The listing builds one solid part. Answer for the finished solid, in the listing's coordinates (mm). A direction names the side the tool comes from. Give positions to 0.01 mm unless a question says otherwise; leave off trailing zeros. Write each loop counter-clockwise with the first axis right and the second up, starting at its lowest first coordinate (ties: lowest second). Pieces come first, ordered by that corner, then holes. Notation, with made-up numbers: (35, 7.5) -> (45, 7.5) arc R26 cw to (45, 34.5) -> close; hole circle Ø10 at (59, 44). An arc over 180 degrees is marked (long way). Write each question's results on one line, items separated by ' | '. Start each with the question number.
from build123d import *

# Parameters (mm, degrees)
EXTRUDE1_DEPTH            = 12.7
F_6_32_TAPPED_HOLE3_D     = 2.7051
SKETCH14_R                = 1.85
CUT_EXTRUDE6_DEPTH        = 24.153833376
F_6_32_TAPPED_HOLE5_D     = 2.7051
F_6_32_TAPPED_HOLE5_DEPTH = 50.8
F_6_32_TAPPED_HOLE5_TIP   = 0.81269403
CUT_EXTRUDE26_DEPTH       = 6
SKETCH25_R                = 5.7
CUT_EXTRUDE27_DEPTH       = 23.907422501
SKETCH26_R                = 8
CUT_EXTRUDE28_DEPTH       = 6


with BuildPart() as part:
    # Sketch1 → Extrude1 (new body)
    with BuildSketch(Plane.XY):
        with BuildLine():
            Line((0, 0), (0, 0.5))
            Line((0, 0.5), (15.5, 0.5))
            Line((15.5, 0.5), (15.5, 4))
            ThreePointArc((15.5, 4), (11.819050527, 4.746581358), (8.719864541, 6.868330393))
            ThreePointArc((8.719864541, 6.868330393), (-11.1, 0), (8.719864541, -6.868330393))
            ThreePointArc((8.719864541, -6.868330393), (11.819050527, -4.746581358), (15.5, -4))
            Line((15.5, -4), (15.5, -0.5))
            Line((15.5, -0.5), (0, -0.5))
            Line((0, -0.5), (0, 0))
        make_face()
    extrude(amount=-EXTRUDE1_DEPTH)

    # #6-32 Tapped Hole3 (through all)
    with Locations(Plane(origin=(-5.656516225, 5.657192254, 0), x_dir=(1, 0, 0), z_dir=(0, 0, 1))):
        with Locations((0, 0), (11.313708479, -0.000676029), (11.31303245, -11.314384508), (-0.000676029, -11.313708479)):
            Hole(F_6_32_TAPPED_HOLE3_D / 2)

    # Sketch14 → Cut-Extrude6 (cut, through all)
    with BuildSketch(Plane.XZ.offset(-0.5)):
        with Locations(Location((13, -3.5, 0), (0, 0, 270))):
            Circle(SKETCH14_R)
    extrude(amount=-CUT_EXTRUDE6_DEPTH, mode=Mode.SUBTRACT)

    # #6-32 Tapped Hole5
    with Locations(Plane(origin=(0, -0.5, 0), x_dir=(-1, 0, 0), z_dir=(0, 1, 0))):
        with Locations((-13, -3.5)):
            Hole(F_6_32_TAPPED_HOLE5_D / 2, depth=F_6_32_TAPPED_HOLE5_DEPTH)
            with Locations((0, 0, -(F_6_32_TAPPED_HOLE5_DEPTH + F_6_32_TAPPED_HOLE5_TIP / 2))):  # 118° drill point
                Cone(0, F_6_32_TAPPED_HOLE5_D / 2, F_6_32_TAPPED_HOLE5_TIP, mode=Mode.SUBTRACT)

    # Sketch24 → Cut-Extrude26 (cut)
    with BuildSketch(Plane(origin=(15.5, 0, 0), x_dir=(0, 0, -1), z_dir=(1, 0, 0))):
        with BuildLine():
            Line((0.2, 4), (6.832300833, 4))
            ThreePointArc((6.832300833, 4), (3.516150417, 6.820400286), (0.2, 4))
        make_face()
    extrude(amount=-CUT_EXTRUDE26_DEPTH, mode=Mode.SUBTRACT)

    # Sketch25 → Cut-Extrude27 (cut, through all)
    with BuildSketch(Plane.XY):
        Circle(SKETCH25_R)
    extrude(amount=-CUT_EXTRUDE27_DEPTH, mode=Mode.SUBTRACT)

    # Sketch26 → Cut-Extrude28 (cut)
    with BuildSketch(Plane.XY):
        Circle(SKETCH26_R)
    extrude(amount=-CUT_EXTRUDE28_DEPTH, mode=Mode.SUBTRACT)


solid = part.part
1. The mould has two halves that part along X. Classify faces 6 (the flat face through (11, -0.5, -6)), 7 (the cylindrical face through (-8, 0, -3)), 8 (the cylindrical face through (11.77, -4.767, -6.261)): pulls with the +X half, pulls with the -X half, needs draft (parallel to the pull), parting line crosses it, or undercut.
2. Consider probe 1 along X at (y, z) = (1.5, -5); probe 2 along X at (y, z) = (-2, -3.5); probe 3 along Y at (x, z) = (-0.75, -4.25). Determine where each line is inside the solid, lowest interval first. Write a range as [from, to].
3. Section D-D (z = -11) is taken. Write down the section's boundary in (x, y), then the cut area to 3 significant figures.
4. Section A-A (y = 3.25) is taken. Write down the section's boundary in (x, z).
5. Each of these flat-tipped pins is pushed along its axis until it touches: pin 1 Ø2.5 at (y, z) = (5, -4.5) entering from +X; pin 2 Ø9 at (x, y) = (0, 0) entering from -Z; pin 3 Ø4 at (x, z) = (4, -3) entering from +Y; pin 4 Ø3.5 at (x, z) = (13, -3.5) entering from +Y. Where does it stop, or does it pass through?
6. Section B-B (x = 0) is taken. Write down the section's boundary in (y, z).
7. Section C-C (z = -3) is taken. Write down the section's boundary in (x, y).
8. A tool of negligible diameter and unlimited length cuts with its end or side. For faces 1 (the flat face through (8, -2, 0)), 2 (the flat face through (11, 0.5, -8)), 3 (the cylindrical face through (7.554, 2.633, -2.958)), 4 (the flat face through (9.5, 5, -3)), 5 (the cylindrical face through (-6.38, 6.8, -7.85)), from which of +Z, -Z, +X, -X, +Y, -Y can it reach the whole face along a straight path? Write none if from no direction.
Results:
1) face 6: needs draft | face 7: undercut | face 8: pulls with the +X half
2) probe 1: x = [-11, -7.86], [7.86, 11.92], [14.08, 15.5] | probe 2: x = [-10.92, -7.75], [7.75, 11.65], [14.35, 15.5] | probe 3: y = [-11.07, -7.96], [7.96, 11.07]
3) outline: (5.68, -0.5) arc R5.7 cw (long way) to (5.68, 0.5) -> (15.5, 0.5) -> (15.5, 4) arc R9.45 cw to (8.72, 6.87) arc R11.1 ccw (long way) to (8.72, -6.87) arc R9.45 cw to (15.5, -4) -> (15.5, -0.5) -> close; hole circle Ø2.71 at (-5.66, -5.66); hole circle Ø2.71 at (-5.66, 5.66); hole circle Ø2.71 at (5.66, -5.66); hole circle Ø2.71 at (5.66, 5.66) | area: 296 mm²
4) outline: (-10.61, -12.7) -> (-4.68, -12.7) -> (-4.68, -6) -> (-7.31, -6) -> (-7.31, 0) -> (-10.61, 0) -> close; (4.68, -12.7) -> (15.5, -12.7) -> (15.5, 0) -> (7.31, 0) -> (7.31, -6) -> (4.68, -6) -> close; hole circle Ø3.7 at (13, -3.5)
5) pin 1: stops at x = 15.5 | pin 2: passes through | pin 3: stops at y = 10.92 | pin 4: stops at y = -0.5
6) outline: (-11.1, -12.7) -> (-5.7, -12.7) -> (-5.7, -6) -> (-8, -6) -> (-8, 0) -> (-11.1, 0) -> close; (5.7, -12.7) -> (11.1, -12.7) -> (11.1, 0) -> (8, 0) -> (8, -6) -> (5.7, -6) -> close
7) outline: (-6.53, -4.62) arc R8 cw to (-6.53, 4.62) arc R1.35 cw (long way) to (-4.62, 6.53) arc R8 cw to (4.62, 6.53) arc R1.35 cw (long way) to (6.53, 4.62) arc R8 cw to (7.98, 0.5) -> (11.22, 0.5) -> (11.22, 4) -> (9.5, 4) -> (9.5, 6.15) arc R9.45 cw to (8.72, 6.87) arc R11.1 ccw (long way) to (8.72, -6.87) arc R9.45 cw to (11.74, -4.78) -> (11.74, -0.5) -> (7.98, -0.5) arc R8 cw to (6.53, -4.62) arc R1.35 cw (long way) to (4.62, -6.53) arc R8 cw to (-4.62, -6.53) arc R1.35 cw (long way) to start; (14.26, -4.08) arc R9.45 cw to (15.5, -4) -> (15.5, -0.5) -> (14.26, -0.5) -> close; (14.78, 0.5) -> (15.5, 0.5) -> (15.5, 4) -> (14.78, 4) -> close
8) face 1: +Z, +X, -X, +Y, -Y | face 2: +Z, -Z, +X | face 3: +Z | face 4: +X | face 5: +Z, -Z
